```python
from build123d import *

# Parameters (mm, degrees)
BOSS_EXTRUDE1_DEPTH = 3
SKETCH2_R           = 4
CUT_EXTRUDE1_DEPTH  = 46.705579528
SKETCH3_R           = 2.05
CUT_EXTRUDE2_DEPTH  = 46.705579528


with BuildPart() as part:
    # Sketch1 → Boss-Extrude1 (new body)
    with BuildSketch(Plane(origin=(0, 0, 0), x_dir=(1, 0, 0), z_dir=(0, 1, 0))):
        with BuildLine():
            Line((0, 12), (32, 12))
            ThreePointArc((32, 12), (44, 0), (32, -12))
            Line((32, -12), (0, -12))
            ThreePointArc((0, -12), (-12, 0), (0, 12))
        make_face()
    extrude(amount=BOSS_EXTRUDE1_DEPTH)

    # Sketch2 → Cut-Extrude1 (cut, through all)
    with BuildSketch(Plane(origin=(0, 3, 0), x_dir=(1, 0, 0), z_dir=(0, 1, 0))):
        with Locations(Location((0, 0, 0), (0, 0, 270))):
            Circle(SKETCH2_R)
        with Locations(Location((16, 0, 0), (0, 0, 270))):
            Circle(SKETCH2_R)
        with Locations(Location((32, 0, 0), (0, 0, 270))):
            Circle(SKETCH2_R)
    extrude(amount=-CUT_EXTRUDE1_DEPTH, mode=Mode.SUBTRACT)

    # Sketch3 → Cut-Extrude2 (cut, through all)
    with BuildSketch(Plane(origin=(0, 3, 0), x_dir=(1, 0, 0), z_dir=(0, 1, 0))):
        with Locations(Location((0, 8, 0), (0, 0, 270))):
            Circle(SKETCH3_R)
        with Locations(Location((5.656854249, 5.656854249, 0), (0, 0, 270))):
            Circle(SKETCH3_R)
        with Locations(Location((8, 0, 0), (0, 0, 270))):
            Circle(SKETCH3_R)
        with Locations(Location((5.656854249, -5.656854249, 0), (0, 0, 270))):
            Circle(SKETCH3_R)
        with Locations(Location((0, -8, 0), (0, 0, 270))):
            Circle(SKETCH3_R)
        with Locations(Location((-5.656854249, -5.656854249, 0), (0, 0, 270))):
            Circle(SKETCH3_R)
        with Locations(Location((-8, 0, 0), (0, 0, 270))):
            Circle(SKETCH3_R)
        with Locations(Location((-5.656854249, 5.656854249, 0), (0, 0, 270))):
            Circle(SKETCH3_R)
        with Locations(Location((26.343145751, -5.656854249, 0), (0, 0, 90))):
            Circle(SKETCH3_R)
        with Locations(Location((32, -8, 0), (0, 0, 90))):
            Circle(SKETCH3_R)
        with Locations(Location((37.656854249, -5.656854249, 0), (0, 0, 90))):
            Circle(SKETCH3_R)
        with Locations(Location((40, 0, 0), (0, 0, 90))):
            Circle(SKETCH3_R)
        with Locations(Location((37.656854249, 5.656854249, 0), (0, 0, 90))):
            Circle(SKETCH3_R)
        with Locations(Location((32, 8, 0), (0, 0, 90))):
            Circle(SKETCH3_R)
        with Locations(Location((26.343145751, 5.656854249, 0), (0, 0, 90))):
            Circle(SKETCH3_R)
        with Locations(Location((24, 0, 0), (0, 0, 90))):
            Circle(SKETCH3_R)
        with Locations(Location((16, 8, 0), (0, 0, 270))):
            Circle(SKETCH3_R)
        with Locations(Location((16, -8, 0), (0, 0, 270))):
            Circle(SKETCH3_R)
    extrude(amount=-CUT_EXTRUDE2_DEPTH, mode=Mode.SUBTRACT)


solid = part.part
```
Geometry check sheet. Reference: the model listing, model coordinates, mm. Round coordinates to 2 decimals unless told otherwise and drop trailing zeros. Loops run counter-clockwise (first coordinate to the right, second up) from the corner with the lowest first, then second, coordinate; pieces in that order, holes last. Notation, with made-up numbers: (21.5, 13.5) - (57.5, 13.5) arc R13 cw to (57.5, 18.5) - close; hole circle Ø9 at (-39, 23). An arc over 180 degrees is marked (long way). Use a Markdown table: item, result.
Q1. Cross-section at D-D on z = 4.5. Record the cut outline in (x, y).
Solutions:
| item | result |
|---|---|
| outline | (-11.12, 0) - (-7.35, 0) - (-7.35, 3) - (-11.12, 3) - close; (-3.96, 0) - (3.96, 0) - (3.96, 3) - (-3.96, 3) - close; (7.35, 0) - (24.65, 0) - (24.65, 3) - (7.35, 3) - close; (28.04, 0) - (35.96, 0) - (35.96, 3) - (28.04, 3) - close; (39.35, 0) - (43.12, 0) - (43.12, 3) - (39.35, 3) - close |
Q2. Cross-section at B-B on z = -8.25. Record the cut outline in (x, y).
Solutions:
| item | result |
|---|---|
| outline | (-8.71, 0) - (-2.03, 0) - (-2.03, 3) - (-8.71, 3) - close; (2.03, 0) - (13.97, 0) - (13.97, 3) - (2.03, 3) - close; (18.03, 0) - (29.97, 0) - (29.97, 3) - (18.03, 3) - close; (34.03, 0) - (40.71, 0) - (40.71, 3) - (34.03, 3) - close |
Q3. Material ranges on line 1 (Z direction, x = 26.5, y = 0.7); line 2 (X direction, y = 1, z = -8); line 3 (Z direction, x = 15, y = 2.85), recorded low to high.
Solutions:
| item | result |
|---|---|
| line 1 | z = -12 to -7.7, -3.61 to 3.61, 7.7 to 12 |
| line 2 | x = -8.94 to -2.05, 2.05 to 13.95, 18.05 to 29.95, 34.05 to 40.94 |
| line 3 | z = -12 to -9.79, -6.21 to -3.87, 3.87 to 6.21, 9.79 to 12 |
Q4. Draft check along X on faces 1 (the cylindrical face through (6.181, 1.521, 0.946)), 2 (the cylindrical face through (44, 1, 0)), 3 (the flat face through (16, 1, -12)). Enter one of: released by +X, released by -X, zero draft, split by the parting line, or undercut.
Solutions:
| item | result |
|---|---|
| face 1 | undercut |
| face 2 | released by +X |
| face 3 | zero draft |
Q5. Cross-section at A-A on x = 16. Record the cut outline in (y, z), plus the area to 3 significant figures.
Solutions:
| item | result |
|---|---|
| outline | (0, -12) - (3, -12) - (3, -10.05) - (0, -10.05) - close; (0, -5.95) - (3, -5.95) - (3, -4) - (0, -4) - close; (0, 4) - (3, 4) - (3, 5.95) - (0, 5.95) - close; (0, 10.05) - (3, 10.05) - (3, 12) - (0, 12) - close |
| area | 23.4 mm2 |
Q6. Go/stop test with flat-tipped pins: P1, Ø3.5, axis at x = 40, z = 0, coming from the +Y side; P2, Ø12, axis at x = 38, z = -3.5, coming from the -Y side. Record where each tip stops, or that it passes through.
Solutions:
| item | result |
|---|---|
| P1 | passes through |
| P2 | stops at y = 0 |
Q7. Cross-section at C-C on y = 2.05. State how many separate pieces and enclosed holes the cut face has, plus the area to 3 significant figures.
Solutions:
| item | result |
|---|---|
| separate pieces | 1 |
| enclosed holes | 21 |
| area | 832 mm2 |
